For this review, take the finished solid that the model builds, in its own axes (mm). A direction names the side the tool comes from. Coordinates: 2 decimals unless noted, no trailing zeros. Order: outer loops, then holes, each group sorted by start corner. A loop starts at its lowest first (then second) coordinate and runs counter-clockwise, first axis right, second up. Notation, with made-up numbers: M 39,2 L 71,2 A12 ccw 71,22 Z; hole C 9,-8.5 d11. An arc over 180 degrees is marked long. Use CSV: the item, a comma, the result in double quotes.
```python
from build123d import *

# Parameters (mm, degrees)
BASE_FLANGE1_DEPTH        = 20
HEM1_DEPTH                = 20
HEM1_2_DEPTH              = 20
SKETCH5_W                 = 8
SKETCH5_H                 = 5
SKETCH5_W_2               = 2
CUT_EXTRUDE4_DEPTH        = 10
M2X0_4_TAPPED_HOLE1_D     = 1.6
M2X0_4_TAPPED_HOLE1_DEPTH = 5.2
M2X0_4_TAPPED_HOLE1_TIP   = 0.480688495


# Read off the part's stored shape, not the designer's step: Hem1
# Sheet-metal steps are written as plain solids
with BuildPart() as part:
    # Sketch1 → Base-Flange1 (new body)
    with BuildSketch(Plane.XY):
        with BuildLine():
            Line((0, 0), (0, 5))
            ThreePointArc((0, 5), (-0.585786438, 6.414213562), (-2, 7))
            Line((-2, 7), (-12.5, 7))
            ThreePointArc((-12.5, 7), (-13.914213562, 6.414213562), (-14.5, 5))
            Line((-14.5, 5), (-14.5, 1))
            Line((-14.5, 1), (-13.5, 1))
            Line((-13.5, 1), (-13.5, 5))
            ThreePointArc((-13.5, 5), (-13.207106781, 5.707106781), (-12.5, 6))
            Line((-12.5, 6), (-2, 6))
            ThreePointArc((-2, 6), (-1.292893219, 5.707106781), (-1, 5))
            Line((-1, 5), (-1, 0))
            Line((-1, 0), (0, 0))
        make_face()
    extrude(amount=BASE_FLANGE1_DEPTH)

    # Hem1 outline → Hem1 (cut)
    with BuildSketch(Plane.XY):
        with BuildLine():
            Line((-13.5, 1), (-13.5, 1.5))
            ThreePointArc((-13.5, 1.5), (-14.236067978, 2.381966011), (-14.5, 3.5))
            Line((-14.5, 3.5), (-14.5, 1))
            Line((-14.5, 1), (-13.5, 1))
        make_face()
    extrude(amount=HEM1_DEPTH, mode=Mode.SUBTRACT)

    # Hem1 2 outline → Hem1 2 (add)
    with BuildSketch(Plane.XY):
        with BuildLine():
            Line((-13.173678907, 5.707368982), (-12.704207344, 4.824421389))
            ThreePointArc((-12.704207344, 4.824421389), (-10.714249049, 2.727442887), (-13.5, 3.5))
            Line((-13.5, 3.5), (-13.5, 1.5))
            ThreePointArc((-13.5, 1.5), (-9.507485574, 3.30668203), (-13.173678907, 5.707368982))
        make_face()
    extrude(amount=HEM1_2_DEPTH)

    # Sketch5 → Cut-Extrude4 (cut)
    with BuildSketch(Plane(origin=(0, 7, 0), x_dir=(1, 0, 0), z_dir=(0, 1, 0))):
        with Locations((-8.5, -10)):
            Rectangle(SKETCH5_W, SKETCH5_H)
        with Locations((-13.5, -10)):
            Rectangle(SKETCH5_W_2, SKETCH5_H)
    extrude(amount=-CUT_EXTRUDE4_DEPTH, mode=Mode.SUBTRACT)

    # M2x0.4 Tapped Hole1
    with Locations(Plane.ZY.offset(1)):
        with Locations((2.5, 3), (17.5, 3)):
            Hole(M2X0_4_TAPPED_HOLE1_D / 2, depth=M2X0_4_TAPPED_HOLE1_DEPTH)
            with Locations((0, 0, -(M2X0_4_TAPPED_HOLE1_DEPTH + M2X0_4_TAPPED_HOLE1_TIP / 2))):  # 118° drill point
                Cone(0, M2X0_4_TAPPED_HOLE1_D / 2, M2X0_4_TAPPED_HOLE1_TIP, mode=Mode.SUBTRACT)


solid = part.part
```
Item 1: For faces 4 (the face through (-0.49, 2.22, 17.67)), 5 (the face through (-4.5, 6.5, 10)), 6 (the face through (-13.5, 4, 4)), 7 (the face through (-7.4, 6.7, 0)), list the 3-axis set-ups (+Z, -Z, +X, -X, +Y, -Y) from which the entire face can be reached by the end or side of a thin tool; tool diameter is ignored.
Solutions:
face 4,"+X"
face 5,"-X, +Y, -Y"
face 6,"+Z, -Z"
face 7,"-Z, +X, -X, +Y, -Y"
Item 2: Add section B-B on x = -8.5. State the section outline as (y, z) points.
Solutions:
outline,"M 6,0 L 7,0 L 7,7.5 L 6,7.5 Z; M 6,12.5 L 7,12.5 L 7,20 L 6,20 Z"
Item 3: Add section D-D on y = 0.5. State the section outline as (x, z) points, and give its area (3 significant figures).
Solutions:
outline,"M -1,0 L 0,0 L 0,20 L -1,20 Z"
area,"20.0 mm^2"
Item 4: Draft analysis for pull direction X (two halves, no side actions). For faces 1 (the face through (-10.69, 2.77, 3.7)), 2 (the face through (-0.5, 0, 9.9)), 3 (the face through (-13.9, 6.43, 3.7)), state which applies: released by +X, released by -X, zero draft, split by the parting line, or undercut.
Solutions:
face 1,"undercut"
face 2,"zero draft"
face 3,"released by -X"
Item 5: Clearance check with flat-ended pins moving along their axes: pin 1 Ø1 at (y, z) = (3, 2.5) entering from +X; pin 2 Ø0.5 at (y, z) = (6.5, 11) entering from -X; pin 3 Ø4 at (y, z) = (5.5, 5.5) entering from -X; pin 4 Ø1.8 at (x, y) = (-12, 3.5) entering from -Z. State where each tip first meets the part, or that it passes through.
Solutions:
pin 1,"x = -9.5"
pin 2,"x = -4.5"
pin 3,"x = -14.5"
pin 4,"through"
Item 6: Add section C-C on z = 9.5. State the section outline as (x, y) points.
Solutions:
outline,"M -4.5,6 L -2,6 A1 cw -1,5 L -1,0 L 0,0 L 0,5 A2 ccw -2,7 L -4.5,7 Z"
Item 7: To check wall thickness, follow line 1 along X through (y, z) = (3.5, 18.5); line 2 along Z through (x, y) = (-12.75, 6.5); line 3 along X through (y, z) = (3, 9). State the ranges of each line that lie inside material, in increasing order. Write a range as [from, to].
Solutions:
line 1,"[-14.5, -13.5], [-10.5, -9.5], [-1, 0]"
line 2,"[0, 7.5], [12.5, 20]"
line 3,"[-1, 0]"
